The listing builds one solid part. Answer for the finished solid, in the listing's coordinates (mm). Round coordinates to 2 decimals unless told otherwise and drop trailing zeros. Write each loop counter-clockwise with the first axis right and the second up, starting at its lowest first coordinate (ties: lowest second). Pieces come first, ordered by that corner, then holes. Notation, with made-up numbers: (60.25, 51.25) -> (80.25, 51.25) arc R8 ccw to (80.25, 56.25) -> close; hole circle Ø6 at (48, 66). An arc over 180 degrees is marked (long way). Write each question's results on one line, items separated by ' | '. Start each with the question number.
```python
from build123d import *

# Parameters (mm, degrees)
SKETCH1_R           = 1.5
BOSS_EXTRUDE1_DEPTH = 10
CUT_EXTRUDE1_DEPTH  = 0.5


with BuildPart() as part:
    # Sketch1 → Boss-Extrude1 (new body)
    with BuildSketch(Plane.XY):
        Circle(SKETCH1_R)
    extrude(amount=BOSS_EXTRUDE1_DEPTH)

    # Sketch3 → Revolve1 (revolve)
    with BuildSketch(Plane(origin=(0, 0, 0), x_dir=(1, 0, 0), z_dir=(0, 1, 0)), mode=Mode.PRIVATE) as revolve1_sk:
        Polygon((-1.5, -10), (-2.5, -11), (0, -11), (0, -10), align=None)
    revolve(revolve1_sk.sketch.rotate(Axis((0, 0, 11), (0, 0, -1)), 180), axis=Axis((0, 0, 11), (0, 0, -1)))

    # Sketch4 → Cut-Extrude1 (cut)
    with BuildSketch(Plane.XY.offset(11)):
        with BuildLine():
            Line((-1.5, 0.37089394), (1.5, 0.37089394))
            ThreePointArc((1.5, 0.37089394), (1.87089394, 0), (1.5, -0.37089394))
            Line((1.5, -0.37089394), (-1.5, -0.37089394))
            ThreePointArc((-1.5, -0.37089394), (-1.87089394, 0), (-1.5, 0.37089394))
        make_face()
    extrude(amount=-CUT_EXTRUDE1_DEPTH, mode=Mode.SUBTRACT)


solid = part.part
```
Q1. The part is cut by section B-B, the plane y = 0. Write down the section's boundary in (x, z), then the cut area to 3 significant figures.
Q2. The part is cut by section A-A, the plane x = 0. Write down the section's boundary in (y, z).
Q3. Each of these flat-tipped pins is pushed along its axis until it touches: pin 1 (0.6 mm diameter, centred on x = -0.5, z = 11, fed in from -Y); pin 2 (1 mm diameter, centred on y = 1, z = 7, fed in from +X); pin 3 (1 mm diameter, centred on y = 1, z = 3, fed in from -X). Where does it stop, or does it pass through?
Q4. Find the intervals of material crossed by line 1 (Y direction, x = 0.05, z = 4.75); line 2 (Z direction, x = 1.75, y = -0.45); line 3 (Z direction, x = -2.05, y = -0.75), in increasing order.
Q5. The part is cut by section C-C, the plane z = 9.75. Write down the section's boundary in (x, y), then the cut area to 3 significant figures.
Q6. Determine the mould class of faces 1 (the flat face through (0, 1, 11)), 2 (the flat face through (0, 0, 0)), 3 (the cylindrical face through (-1.5, 0.07, 4.93)) for opening direction Z: pulls with the +Z half, pulls with the -Z half, needs draft (parallel to the pull), parting line crosses it, or undercut.
Answers follow:
1) outline: (-2.5, 11) -> (-1.5, 10) -> (-1.5, 0) -> (1.5, 0) -> (1.5, 10) -> (2.5, 11) -> (1.87, 11) -> (1.87, 10.5) -> (-1.87, 10.5) -> (-1.87, 11) -> close | area: 32.1 mm^2
2) outline: (-2.5, 11) -> (-1.5, 10) -> (-1.5, 0) -> (1.5, 0) -> (1.5, 10) -> (2.5, 11) -> (0.37, 11) -> (0.37, 10.5) -> (-0.37, 10.5) -> (-0.37, 11) -> close
3) pin 1: y = -2.49 | pin 2: x = 1.41 | pin 3: x = -1.41
4) line 1: -1.5 to 1.5 | line 2: 10.31 to 11 | line 3: 10.68 to 11
5) outline: circle Ø3 at (0, 0) | area: 7.07 mm^2
6) face 1: pulls with the +Z half | face 2: pulls with the -Z half | face 3: needs draft
